```python
from build123d import *

# Parameters (mm, degrees)
F0_W      = 132
F0_H      = 109
F0_R      = 3.5
F0_R_2    = 2
F1_DEPTH  = 1
F2_W      = 132
F2_H      = 109
F2_R      = 3.5
F2_R_2    = 2
F2_R_3    = 2.5
F3_DEPTH  = 1
F4_R      = 2.5
F4_R_2    = 2
F5_DEPTH  = 1
F6_W      = 9
F6_H      = 9.5
F7_DEPTH  = 3
F8_R      = 3
F8_R_2    = 2
F8_R_3    = 3.5
F8_W      = 28
F8_H      = 16
F8_R_4    = 1.25
F9_DEPTH  = 2
F10_W     = 4
F10_H     = 9.5
F9_FACE_W = 28
F9_FACE_H = 16
F9_FACE_R = 1.25
F11_DEPTH = 6
F12_R     = 0.75
F13_DEPTH = 7
F14_W     = 28
F14_H     = 16
F14_R     = 1.25
F15_DEPTH = 6


# Not quite as in the source:
# - a feature names something its author has since deleted; it is built from what else it names


with BuildPart() as f1:
    # F0 (on Top) → F1 (new body)
    with BuildSketch(Plane.XY):
        with Locations((66, 54.5)):
            Rectangle(F0_W, F0_H)
        with Locations((5, 38)):
            Circle(F0_R, mode=Mode.SUBTRACT)
        with Locations((125, 22)):
            Circle(F0_R, mode=Mode.SUBTRACT)
        with Locations((66, 35)):
            Circle(F0_R_2, mode=Mode.SUBTRACT)
        with Locations((118, 40)):
            Circle(F0_R_2, mode=Mode.SUBTRACT)
        with Locations((5, 86)):
            Circle(F0_R_2, mode=Mode.SUBTRACT)
        with Locations((118, 68)):
            Circle(F0_R_2, mode=Mode.SUBTRACT)
        with Locations((67, 83)):
            Circle(F0_R_2, mode=Mode.SUBTRACT)
        with Locations((125, 91)):
            Circle(F0_R_2, mode=Mode.SUBTRACT)
    extrude(amount=F1_DEPTH)

    # F2 (on face) → F3 (join)
    with BuildSketch(Plane.XY.offset(1)):
        with Locations((66, 54.5)):
            Rectangle(F2_W, F2_H)
        with Locations((5, 38)):
            Circle(F2_R, mode=Mode.SUBTRACT)
        with Locations((125, 22)):
            Circle(F2_R, mode=Mode.SUBTRACT)
        with Locations((66, 35)):
            Circle(F2_R_2, mode=Mode.SUBTRACT)
        with Locations((118, 40)):
            Circle(F2_R_2, mode=Mode.SUBTRACT)
        with Locations((5, 86)):
            Circle(F2_R_2, mode=Mode.SUBTRACT)
        with Locations((118, 68)):
            Circle(F2_R_2, mode=Mode.SUBTRACT)
        with Locations((67, 83)):
            Circle(F2_R_2, mode=Mode.SUBTRACT)
        with Locations((125, 91)):
            Circle(F2_R_2, mode=Mode.SUBTRACT)
        with Locations((125, 22)):
            Circle(F2_R)
        with Locations((125, 22)):
            Circle(F2_R_3, mode=Mode.SUBTRACT)
        with Locations((5, 38)):
            Circle(F2_R)
        with Locations((5, 38)):
            Circle(F2_R_3, mode=Mode.SUBTRACT)
    extrude(amount=F3_DEPTH)

    # F4 (on face) → F5 (join)
    with BuildSketch(Plane.XY.offset(2)):
        Polygon((14, 102), (14, 109), (0, 109), (0, 0), (132, 0), (132, 109), (26.5, 109), (26.5, 102), align=None)
        with Locations((5, 38)):
            Circle(F4_R, mode=Mode.SUBTRACT)
        with Locations((125, 22)):
            Circle(F4_R, mode=Mode.SUBTRACT)
        with Locations((66, 35)):
            Circle(F4_R_2, mode=Mode.SUBTRACT)
        with Locations((118, 40)):
            Circle(F4_R_2, mode=Mode.SUBTRACT)
        with Locations((5, 86)):
            Circle(F4_R_2, mode=Mode.SUBTRACT)
        with Locations((118, 68)):
            Circle(F4_R_2, mode=Mode.SUBTRACT)
        with Locations((67, 83)):
            Circle(F4_R_2, mode=Mode.SUBTRACT)
        with Locations((125, 91)):
            Circle(F4_R_2, mode=Mode.SUBTRACT)
    extrude(amount=F5_DEPTH)

    # F6 (on face) → F7 (cut)
    with BuildSketch(Plane.XY.offset(3)):
        with Locations((107, 104.25)):
            Rectangle(F6_W, F6_H)
    extrude(amount=-F7_DEPTH, mode=Mode.SUBTRACT)

    # F8 (on face) → F9 (join)
    with BuildSketch(Plane.XY.offset(3)):
        Polygon((14, 102), (14, 109), (10, 109), (10, 98), (30.5, 98), (30.5, 109), (26.5, 109), (26.5, 102), align=None)
        Polygon((102.5, 109), (98.5, 109), (98.5, 92), (115.5, 92), (115.5, 109), (111.5, 109), (111.5, 99.5), (102.5, 99.5), align=None)
        with Locations((67, 83)):
            Circle(F8_R)
        with Locations((67, 83)):
            Circle(F8_R_2, mode=Mode.SUBTRACT)
        with Locations((66, 35)):
            Circle(F8_R_3)
        with Locations((66, 35)):
            Circle(F8_R_2, mode=Mode.SUBTRACT)
        with Locations((118, 68)):
            Circle(F8_R_3)
        with Locations((118, 68)):
            Circle(F8_R_2, mode=Mode.SUBTRACT)
        with Locations((118, 40)):
            Circle(F8_R_3)
        with Locations((118, 40)):
            Circle(F8_R_2, mode=Mode.SUBTRACT)
        with Locations((29, 18)):
            Rectangle(F8_W, F8_H)
        with Locations((18, 23)):
            Circle(F8_R_4, mode=Mode.SUBTRACT)
        with Locations((40, 13)):
            Circle(F8_R_4, mode=Mode.SUBTRACT)
    extrude(amount=F9_DEPTH)

    # F10 (on face) + F9_face (on face) → F11 (join)
    with BuildSketch(Plane.XY.offset(5)):
        with Locations((100.5, 104.25)):
            Rectangle(F10_W, F10_H)
        with Locations((113.5, 104.25)):
            Rectangle(F10_W, F10_H)
    with BuildSketch(Plane(origin=(67, 83, 5), x_dir=(1, 0, 0), z_dir=(0, 0, 1))):
        with Locations((-38, -65)):
            Rectangle(F9_FACE_W, F9_FACE_H)
        with Locations((-49, -60)):
            Circle(F9_FACE_R, mode=Mode.SUBTRACT)
        with Locations((-27, -70)):
            Circle(F9_FACE_R, mode=Mode.SUBTRACT)
    extrude(amount=F11_DEPTH)

    # F12 (on face) → F13 (cut)
    with BuildSketch(Plane(origin=(0, 99.5, 0), x_dir=(-1, 0, 0), z_dir=(0, 1, 0))):
        with Locations((-107, 3)):
            Circle(F12_R)
    extrude(amount=-F13_DEPTH, mode=Mode.SUBTRACT)

    # F14 (on face) → F15 (join)
    with BuildSketch(Plane.XY.offset(11)):
        with Locations((29, 18)):
            Rectangle(F14_W, F14_H)
        with Locations((40, 13)):
            Circle(F14_R, mode=Mode.SUBTRACT)
        with Locations((18, 23)):
            Circle(F14_R, mode=Mode.SUBTRACT)
    extrude(amount=F15_DEPTH)


solid = f1.part
```
Model file for the job. Use its own axes, mm. A direction names the side the tool comes from. Coordinates: 2 decimals unless noted, no trailing zeros. Order: outer loops, then holes, each group sorted by start corner. A loop starts at its lowest first (then second) coordinate and runs counter-clockwise, first axis right, second up. Notation, with made-up numbers: M 8.25,68 L 24.25,68 A30 cw 24.25,94 Z; hole C -6,5.25 d3. An arc over 180 degrees is marked long. Answer as CSV lines item,"result".
(1) Pull direction X, two halves, no side cores. Call faces 4 (the flat face through (100, 99.5, 8)), 5 (the flat face through (111.5, 104, 6)), 6 (the flat face through (0, 55, 1)): +X half, -X half, draft (parallel to the pull), parting line (faces both ways), or undercut.
Geometry says:
face 4,"draft"
face 5,"undercut"
face 6,"-X half"
(2) Wall check: line 1 along Y through (x, z) = (125, 0.8); line 2 along Y through (x, z) = (125, 1.45); line 3 along Z through (x, y) = (118.5, 72). Give the ranges that are in metal, low to high.
Geometry says:
line 1,"y = 0 to 18.5, 25.5 to 89, 93 to 109"
line 2,"y = 0 to 19.5, 24.5 to 89, 93 to 109"
line 3,"z = 0 to 3"
(3) Band-saw the part on C-C, the plane y = 17. List the corners of the cut face in (x, z), then the cut area to 3 significant figures.
Geometry says:
outline,"M 0,0 L 132,0 L 132,3 L 43,3 L 43,17 L 15,17 L 15,3 L 0,3 Z"
area,"788 mm2"
(4) Band-saw the part on B-B, the plane z = 14.5. List the corners of the cut face in (x, y), then the cut area to 3 significant figures.
Geometry says:
outline,"M 15,10 L 43,10 L 43,26 L 15,26 Z; hole C 18,23 d2.5; hole C 40,13 d2.5"
area,"438 mm2"
(5) Band-saw the part on A-A, the plane y = 68. List the corners of the cut face in (x, z).
Geometry says:
outline,"M 0,0 L 116,0 L 116,5 L 114.5,5 L 114.5,3 L 0,3 Z; M 120,0 L 132,0 L 132,3 L 121.5,3 L 121.5,5 L 120,5 Z"
(6) 3-axis set-ups, long thin cutter, end or side, ignore diameter. For faces 1 (the flat face through (98.5, 102, 6)), 2 (the flat face through (127, 20, 1)), 3 (the flat face through (14, 105, 3)): which of +Z, -Z, +X, -X, +Y, -Y reach the whole face in a straight line?
Geometry says:
face 1,"+Z, +Y, -Y"
face 2,"-Z"
face 3,"+Z, +Y"
(7) Flat gauge pins, fed straight in: pin 1 (0.8 mm diameter, centred on x = 17.5, y = 23.5, fed in from +Z); pin 2 (12 mm diameter, centred on x = 20, y = 104, fed in from +Z); pin 3 (0.6 mm diameter, centred on x = 106, z = 3.5, fed in from -Y); pin 4 (4 mm diameter, centred on x = 91, z = 5.5, fed in from -Y). Where does each tip first touch, or does it go through?
Geometry says:
pin 1,"stops at z = 3"
pin 2,"stops at z = 5"
pin 3,"stops at y = 92"
pin 4,"passes through"
